Autodesk Inventor part; units mm, degrees
ref_plane "YZ Plane" through (0, 0, 0) normal (1, 0, 0) x (0, 1, 0)
ref_plane "XZ Plane" through (0, 0, 0) normal (0, 1, 0) x (-1, 0, 0)
ref_plane "XY Plane" through (0, 0, 0) normal (0, 0, 1) x (1, 0, 0)
sketch "Sketch1" plane through (0, 0, 0) normal (0, 1, 0) x (-1, 0, 0)
  arc A0 (44.7326, -45.0693) -> (44.7326, 45.0693) centre (0, 0) ccw
  line L0 (44.6636, -43.1846) -> (57.3636, -43.1846)
  line L1 (57.3636, -43.1846) -> (57.3636, -82.5546)
  line L2 (57.3636, -82.5546) -> (44.6636, -82.5546)
  line L3 (44.6636, -82.5546) -> (44.6636, -43.1846)
  line L4 (44.7326, -53.6471) -> (44.7326, 53.6471)
  arc A1 (44.7326, -53.6471) -> (44.7326, 53.6471) centre (0, 0) ccw
  point P0 (54.901, -43.1846)
  point P1 (46.5547, -43.1846)
  dimension "d0" = 63.5
  dimension "d2" = 12.7
  dimension "d3" = 39.37
extrude "Extrusion1" add sketch "Sketch1" along normal blind 3.175 contours L4 L0 A0 | A0 L0 A1 L4 | L4 A1 L0 L1 L2 L3 | A0 L4 A1 L0 picked at (44.9379, -44.2344)
sketch "Sketch2" plane through (0, 3.175, 0) normal (0, 1, 0) x (1, 0, 0)
  line L0 (-57.3636, 82.5546) -> (-57.3636, 43.1846)
  line L1 (-44.6636, 82.5546) -> (-57.3636, 82.5546)
  line L2 (-46.5547, 43.1846) -> (-44.6636, 43.1846)
  line L3 (-44.6636, 43.1846) -> (-44.6636, 82.5546)
  line L4 (-57.3636, 43.1846) -> (-54.901, 43.1846)
  arc A0 (-54.901, 43.1846) -> (-44.7326, -53.6471) centre (0, 0) ccw
  line L5 (-44.7326, -53.6471) -> (-44.7326, -45.0693)
  arc A1 (-46.5547, 43.1846) -> (-44.7326, -45.0693) centre (0, 0) ccw
  point P0 (-51.0136, 46.9946)
  point P1 (-51.0136, 78.7446)
  dimension "d6" = 12.7
  dimension "d7" = 6.35
  dimension "d8" = 6.35
  dimension "d9" = 31.75
  dimension "d10" = 39.37
  dimension "d11" = 3.81
hole "Hole1" at (-51.0136, 3.175, -46.9946) at (-51.0136, 3.175, -78.7446) direction (0, -1, 0) diameter 6.35 depth 19.05 tip angle 118
properties part number "grabber"
Verification items for the finished model (mm, model axes). A direction names the side the tool comes from. Give positions to 0.01 mm unless a question says otherwise; leave off trailing zeros. Order: outer loops, then holes, each group sorted by start corner. A loop starts at its lowest first (then second) coordinate and runs counter-clockwise, first axis right, second up. Notation, with made-up numbers: M -14,73.5 L -3,73.5 A5 ccw -3,78.5 Z; hole C -3.5,77.5 d1. An arc over 180 degrees is marked long. Answer as a JSON object with one key per item and string values. Group by question number.
1) Depth check by flat-ended pin: pin 1 Ø0.6 at (x, y) = (-45.5, 1.5) entering from +Z; pin 2 Ø1 at (y, z) = (1, -68) entering from -X; pin 3 Ø1 at (y, z) = (1, 11.5) entering from -X; pin 4 Ø4 at (x, z) = (-51.01, -46.99) entering from -Y. Enter the tip coordinate at first touch or a pass-through.
2) Cross-section at D-D (z = -24). Enter the section's corners in (x, y) (3 decimals).
3) Mould release check, pull along Z, two halves, no side actions. Record for faces 1 (the face through (-51, 2, -82.555)), 2 (the face through (-53.7, 1.6, -45.3)), 3 (the face through (-57, 0, -29)), 4 (the face through (-63.47, 1.57, 1.99)): released by +Z, released by -Z, zero draft, split by the parting line, or undercut.
4) Access from +Z, -Z, +X, -X, +Y, -Y to the whole of each face (thin tool, end or side, straight path). Record for faces 5 (the face through (-51.967, 1.565, -75.716)), 6 (the face through (-57.364, 2, -63)).
5) Cross-section at A-A (z = -49). Enter the section's corners in (x, y) (3 decimals), then the cut area to 3 significant figures.
6) Cross-section at B-B (y = 2.2). Enter the section's corners in (x, z) (3 decimals), then the cut area to 3 significant figures.
7) Cross-section at C-C (x = -61.25). Enter the section's corners in (y, z) (3 decimals).
8) Scan lines: line 1 along Z through (x, y) = (-55.5, 1.6); line 2 along Z through (x, y) = (-55.25, 2); line 3 along Z through (x, y) = (-53.75, 1.2). Record each from-to range of solid material in increasing order. Write a range as [from, to].
Result sheet:
{
 "1": {"pin 1": "stops at z = 53.25", "pin 2": "stops at x = -57.36", "pin 3": "stops at x = -68.98", "pin 4": "passes through"},
 "2": {"outline": "M -65.597,0 L -58.79,0 L -58.79,3.175 L -65.597,3.175 Z"},
 "3": {"face 1": "released by -Z", "face 2": "undercut", "face 3": "zero draft", "face 4": "undercut"},
 "4": {"face 5": "+Y, -Y", "face 6": "-Z, -X, +Y, -Y"},
 "5": {"outline": "M -57.364,0 L -53.475,0 L -53.475,3.175 L -57.364,3.175 Z; M -48.552,0 L -44.664,0 L -44.664,3.175 L -48.552,3.175 Z", "area": "24.7 mm2"},
 "6": {"outline": "M -57.364,-82.555 L -44.664,-82.555 L -44.664,-43.185 L -46.555,-43.185 A63.5 cw -44.733,45.069 L -44.733,53.647 A69.85 ccw -54.901,-43.185 L -57.364,-43.185 Z; hole C -51.014,-78.745 d6.35; hole C -51.014,-46.995 d6.35", "area": "1,090 mm2"},
 "7": {"outline": "M 0,-33.578 L 3.175,-33.578 L 3.175,-16.754 L 0,-16.754 Z; M 0,16.754 L 3.175,16.754 L 3.175,33.578 L 0,33.578 Z"},
 "8": {"line 1": "z = [-82.55, -43.18], [-42.41, -30.85], [30.85, 42.41]", "line 2": "z = [-82.55, -43.18], [-42.74, -31.3], [31.3, 42.74]", "line 3": "z = [-82.55, -80.35], [-77.13, -48.6], [-45.38, -33.81], [33.81, 44.61]"}
}
